Autodesk Inventor part; units mm, degrees
ref_plane "YZ Plane" through (0, 0, 0) normal (1, 0, 0) x (0, 1, 0)
ref_plane "XZ Plane" through (0, 0, 0) normal (0, 1, 0) x (-1, 0, 0)
ref_plane "XY Plane" through (0, 0, 0) normal (0, 0, 1) x (1, 0, 0)
sketch "スケッチ1" plane through (0, 0, 0) normal (0, 0, 1) x (1, 0, 0)
  line L0 (-19, -18) -> (19, -18)
  line L1 (19, -18) -> (19, 18)
  line L2 (19, 18) -> (-19, 18)
  line L3 (-19, 18) -> (-19, -18)
  line L4 (-19, -18) -> (19, 18) construction
  line L5 (19, -18) -> (-19, 18) construction
  point P0 (0, 0)
  dimension "d0" = 38
  dimension "d1" = 36
extrude "押し出し1" add sketch "スケッチ1" along normal blind 5
chamfer "面取り1" distance 2 angle 45 8 edges at (0, 18, 5) (19, 0, 5) (0, -18, 5) (-19, 0, 5) (19, -18, 2.5) (-19, -18, 2.5) (-19, 18, 2.5) (19, 18, 2.5)
sketch "スケッチ2" plane through (0, 0, 5) normal (0, 0, 1) x (1, 0, 0)
  line L0 (-19, -18) -> (19, -18)
  line L1 (19, -18) -> (19, 18)
  line L2 (-16, -13) -> (15, -13)
  line L3 (15, -13) -> (15, 3)
  line L4 (15, 3) -> (-16, 3)
  line L5 (-16, 3) -> (-16, -13)
  line L6 (-16, -13) -> (15, 3) construction
  line L7 (15, -13) -> (-16, 3) construction
  point P0 (0, 0)
  point P1 (-0.5, -5)
  dimension "d4" = 31
  dimension "d5" = 16
  dimension "d6" = 5
  dimension "d7" = 4
hole "穴1" at (-16, 3, 5) at (-16, -13, 5) at (15, -13, 5) at (15, 3, 5) direction (0, 0, -1) diameter 3.2 depth 6 counterbore diameter 6.5 counterbore depth 2
sketch "スケッチ3" plane through (0, 0, 0) normal (0, 0, -1) x (-1, 0, 0)
  line L0 (19, 16) -> (19, -16)
  line L1 (-17, 18) -> (17, 18)
  point P0 (0, 0)
  point P1 (-7, 10.5)
  point P2 (7, 10.5)
  dimension "d18" = 7.5
  dimension "d19" = 12
  dimension "d20" = 14
hole "穴2" at (7, 10.5, 0) at (-7, 10.5, 0) direction (0, 0, 1) diameter 6.5 depth 3
properties part number "Print_Parts_S2"
Verification items for the finished model (mm, model axes). A direction names the side the tool comes from. Coordinates: 2 decimals unless noted, no trailing zeros. Order: outer loops, then holes, each group sorted by start corner. A loop starts at its lowest first (then second) coordinate and runs counter-clockwise, first axis right, second up. Notation, with made-up numbers: M 67.5,86 L 113.5,86 A28 cw 113.5,110 Z; hole C 7.25,37 d10. An arc over 180 degrees is marked long. One line per item, written item: value. Start each with the question number.
Item 1: Sectioned sample at C-C (z = 0.55). Enter the section's corners in (x, y), then the cut area to 3 significant figures.
Item 2: Sectioned sample at D-D (y = -13). Enter the section's corners in (x, z).
Item 3: Sectioned sample at B-B (y = 10.5). Enter the section's corners in (x, z), then the cut area to 3 significant figures.
Item 4: Scan lines: probe 1 along Y at (x, z) = (15, 0.95); probe 2 along Y at (x, z) = (14, 3.05); probe 3 along X at (y, z) = (10.5, 0.8). Record each from-to range of solid material in increasing order.
Item 5: Access from +Z, -Z, +X, -X, +Y, -Y to the whole of each face (thin tool, end or side, straight path). Record for faces 1 (the cylindrical face through (6.857, 7.253, 1.521)), 2 (the flat face through (-14.5, -11.5, 3)), 3 (the flat face through (0, 18, 1)).
Item 6: Gauge pin test, flat ends, axial feed: pin 1 (4 mm diameter, centred on x = 15, y = 3, fed in from +Z); pin 2 (1.9 mm diameter, centred on x = -16, y = -13, fed in from +Z); pin 3 (2 mm diameter, centred on x = 7, y = 10, fed in from -Z). Record the tip position at first contact, or that the pin passes through.
Item 7: Mould release check, pull along Y, two halves, no side actions. Record for faces 4 (the flat face through (-18, 17, 1)), 5 (the flat face through (16.4, 1.6, 3)), 6 (the flat face through (0, 0, 0)): released by +Y, released by -Y, zero draft, split by the parting line, or undercut.
Item 8: Sectioned sample at A-A (x = -16). Enter the section's corners in (y, z).
Conclusion:
1. outline: M -19,-16 L -17,-18 L 17,-18 L 19,-16 L 19,16 L 17,18 L -17,18 L -19,16 Z; hole C -16,-13 d3.2; hole C -16,3 d3.2; hole C -7,10.5 d6.5; hole C 7,10.5 d6.5; hole C 15,-13 d3.2; hole C 15,3 d3.2
1. area: 1,260 mm^2
2. outline: M -19,0 L -17.6,0 L -17.6,3 L -19,3 Z; M -14.4,0 L 13.4,0 L 13.4,3 L 11.75,3 L 11.75,5 L -12.75,5 L -12.75,3 L -14.4,3 Z; M 16.6,0 L 19,0 L 19,3 L 18.25,3.75 L 18.25,3 L 16.6,3 Z
3. outline: M -19,0 L -10.25,0 L -10.25,3 L -3.75,3 L -3.75,0 L 3.75,0 L 3.75,3 L 10.25,3 L 10.25,0 L 19,0 L 19,3 L 17,5 L -17,5 L -19,3 Z
3. area: 147 mm^2
4. probe 1: y = -18 to -14.6, -11.4 to 1.4, 4.6 to 18
4. probe 2: y = -17.95 to -16.09, -9.91 to -0.09, 6.09 to 17.95
4. probe 3: x = -19 to -10.25, -3.75 to 3.75, 10.25 to 19
5. face 1: -Z
5. face 2: +Z
5. face 3: +Z, -Z, +X, -X, +Y
6. pin 1: stops at z = 3
6. pin 2: passes through
6. pin 3: stops at z = 3
7. face 4: released by +Y
7. face 5: undercut
7. face 6: zero draft
8. outline: M -18,0 L -14.6,0 L -14.6,3 L -16.25,3 L -16.25,4.75 L -18,3 Z; M -11.4,0 L 1.4,0 L 1.4,3 L -0.25,3 L -0.25,5 L -9.75,5 L -9.75,3 L -11.4,3 Z; M 4.6,0 L 18,0 L 18,3 L 16,5 L 6.25,5 L 6.25,3 L 4.6,3 Z
